```python
from build123d import *

# Parameters (mm, degrees)
SKETCH1_R           = 14.5
SKETCH1_R_2         = 12.5
BOSS_EXTRUDE1_DEPTH = 150
SKETCH2_R           = 2.25
CUT_EXTRUDE1_DEPTH  = 152.395178259
CIRPATTERN1_COUNT   = 4


with BuildPart() as part:
    # Sketch1 → Boss-Extrude1 (new body)
    with BuildSketch(Plane(origin=(0, 0, 0), x_dir=(1, 0, 0), z_dir=(0, 1, 0))):
        with Locations(Location((0, 0, 0), (0, 0, 270))):
            Circle(SKETCH1_R)
        with Locations(Location((0, 0, 0), (0, 0, 270))):
            Circle(SKETCH1_R_2, mode=Mode.SUBTRACT)
    extrude(amount=BOSS_EXTRUDE1_DEPTH)

    # Sketch2 → Cut-Extrude1 (cut, symmetric)
    with BuildSketch(Plane.XY):
        with Locations((0, 140)):
            Circle(SKETCH2_R)
        with Locations((0, 10)):
            Circle(SKETCH2_R)
    cut_extrude1 = extrude(amount=CUT_EXTRUDE1_DEPTH, both=True, mode=Mode.SUBTRACT)

    # CirPattern1: Cut-Extrude1 ×4 about axis
    cirpattern1_axis = Axis((0, 150, 0), (0, -1, 0))
    for i in range(1, CIRPATTERN1_COUNT):
        add(cut_extrude1.rotate(cirpattern1_axis, i * 360 / CIRPATTERN1_COUNT), mode=Mode.SUBTRACT)


solid = part.part
```
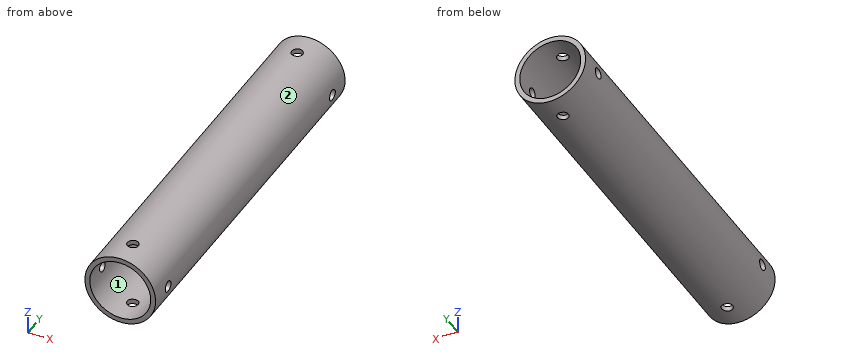
The listing builds one solid part. Answer for the finished solid, in the listing's coordinates (mm). Face numbers are marked on the shaded views. Coordinates: 2 decimals unless noted, no trailing zeros. Write each loop counter-clockwise with the first axis right and the second up, starting at its lowest first coordinate (ties: lowest second). Pieces come first, ordered by that corner, then holes.
Q1. The mould has two halves that part along Z. Classify the marked faces 1 and 2: released by +Z, released by -Z, zero draft, split by the parting line, or undercut.
Returned:
face 1: undercut
face 2: split by the parting line
Q2. Section A-A, the plane z = 0 is taken. Write down the section's boundary in (x, y), then the cut area to 3 significant figures.
Returned:
outline: (-14.5, 0) - (-12.5, 0) - (-12.5, 7.75) - (-14.5, 7.75) - close; (-14.5, 12.25) - (-12.5, 12.25) - (-12.5, 137.75) - (-14.5, 137.75) - close; (-14.5, 142.25) - (-12.5, 142.25) - (-12.5, 150) - (-14.5, 150) - close; (12.5, 0) - (14.5, 0) - (14.5, 7.75) - (12.5, 7.75) - close; (12.5, 12.25) - (14.5, 12.25) - (14.5, 137.75) - (12.5, 137.75) - close; (12.5, 142.25) - (14.5, 142.25) - (14.5, 150) - (12.5, 150) - close
area: 564 mm2
Q3. Given P1, Ø2.5, axis at x = 0, y = 10, coming from the +Z side; P2, Ø5, axis at y = 83, z = -5, coming from the -X side; P3, Ø2, axis at x = 5.5, y = 131.5, coming from the +Z side; P4, Ø1.5, axis at x = 5, y = 40, coming from the +Z side, each flat-ended and moving along its own axis, determine where each tip first touches the part or whether it passes through.
Returned:
P1: passes through
P2: stops at x = -14.28
P3: stops at z = 13.78
P4: stops at z = 13.86
Q4. Section B-B, the plane x = 0 is taken. Write down the section's boundary in (y, z), then the cut area to 3 significant figures.
Returned:
outline: (0, -14.5) - (7.75, -14.5) - (7.75, -12.5) - (0, -12.5) - close; (0, 12.5) - (7.75, 12.5) - (7.75, 14.5) - (0, 14.5) - close; (12.25, -14.5) - (137.75, -14.5) - (137.75, -12.5) - (12.25, -12.5) - close; (12.25, 12.5) - (137.75, 12.5) - (137.75, 14.5) - (12.25, 14.5) - close; (142.25, -14.5) - (150, -14.5) - (150, -12.5) - (142.25, -12.5) - close; (142.25, 12.5) - (150, 12.5) - (150, 14.5) - (142.25, 14.5) - close
area: 564 mm2
Q5. Section C-C, the plane y = 140 is taken. Write down the section's boundary in (x, z), then the cut area to 3 significant figures.
Returned:
outline: (-14.32, -2.25) arc R14.5 ccw to (-2.25, -14.32) - (-2.25, -12.3) arc R12.5 cw to (-12.3, -2.25) - close; (-14.32, 2.25) - (-12.3, 2.25) arc R12.5 cw to (-2.25, 12.3) - (-2.25, 14.32) arc R14.5 ccw to start; (2.25, -14.32) arc R14.5 ccw to (14.32, -2.25) - (12.3, -2.25) arc R12.5 cw to (2.25, -12.3) - close; (2.25, 12.3) arc R12.5 cw to (12.3, 2.25) - (14.32, 2.25) arc R14.5 ccw to (2.25, 14.32) - close
area: 133 mm2
Q6. Find the intervals of material crossed by line 1 along Y through (x, z) = (-14, 0); line 2 along Z through (x, y) = (13.35, 140); line 3 along Z through (x, y) = (-13.4, 140), in increasing order.
Returned:
line 1: y = 0 to 7.75, 12.25 to 137.75, 142.25 to 150
line 2: z = -5.66 to -2.25, 2.25 to 5.66
line 3: z = -5.54 to -2.25, 2.25 to 5.54
Q7. Section D-D, the plane z = -9.75 is taken. Write down the section's boundary in (x, y).
Returned:
outline: (-10.73, 0) - (-7.82, 0) - (-7.82, 150) - (-10.73, 150) - close; (7.82, 0) - (10.73, 0) - (10.73, 150) - (7.82, 150) - close
